Build history of the part. All positions in model axes, mm. A direction names the side the tool comes from. Coordinates: 2 decimals unless noted, no trailing zeros. Write each loop counter-clockwise with the first axis right and the second up, starting at its lowest first coordinate (ties: lowest second). Pieces come first, ordered by that corner, then holes.
from build123d import *

# Parameters (mm, degrees)
BOSS_EXTRUDE1_DEPTH = 6


with BuildPart() as part:
    # Sketch1 → Boss-Extrude1 (new body)
    with BuildSketch(Plane.XY):
        with BuildLine():
            Line((-18.687702572, 18.729195928), (-15.687702572, 18.729195928))
            Line((-15.687702572, 18.729195928), (-15.687702572, 6.729195928))
            Line((-15.687702572, 6.729195928), (-9.687702572, 6.729195928))
            Line((-9.687702572, 6.729195928), (-9.687702572, 12.729195928))
            Line((-9.687702572, 12.729195928), (-6.556235979, 14.903596974))
            ThreePointArc((-6.556235979, 14.903596974), (-2.418100544, 16.566329788), (2.031378501, 16.264698373))
            Line((2.031378501, 16.264698373), (3.503651069, 15.82124278))
            ThreePointArc((3.503651069, 15.82124278), (6.627191746, 15.399192613), (9.726940979, 15.970320798))
            Line((9.726940979, 15.970320798), (14.488027768, 17.656969749))
            Line((14.488027768, 17.656969749), (14.488027768, 4.729195928))
            Line((14.488027768, 4.729195928), (20.488027768, 4.729195928))
            Line((20.488027768, 4.729195928), (20.488027768, 12.729195928))
            Line((20.488027768, 12.729195928), (26.488027768, 12.729195928))
            Line((26.488027768, 12.729195928), (26.488027768, -3.270804072))
            Line((26.488027768, -3.270804072), (3.231231788, -3.270804072))
            Line((3.231231788, -3.270804072), (3.231231788, -9.270804072))
            Line((3.231231788, -9.270804072), (-18.687702572, -9.270804072))
            Line((-18.687702572, -9.270804072), (-18.687702572, 18.729195928))
        make_face()
    extrude(amount=BOSS_EXTRUDE1_DEPTH)


solid = part.part
(1) Slice it at D-D, the plane x = -11. List the corners of the cut face in (y, z), and give its area (3 significant figures).
(2) Slice it at A-A, the plane y = 10.25. List the corners of the cut face in (x, z), and give its area (3 significant figures).
(3) 3-axis set-ups, long thin cutter, end or side, ignore diameter. For faces 4 (the flat face through (26.488, 5, 3)), 5 (the flat face through (-1, 5, 6)), 6 (the flat face through (23, 12.729, 3)), 7 (the flat face through (15, -3.271, 3)), 8 (the flat face through (2.757, 16.046, 2.958)): which of +Z, -Z, +X, -X, +Y, -Y reach the whole face in a straight line?
(4) Flat gauge pins, fed straight in: P1, Ø3, axis at x = 23, z = 3.5, coming from the +Y side; P2, Ø3, axis at x = 18.5, z = 3, coming from the +Y side; P3, Ø1.5, axis at x = 17.5, z = 3, coming from the -Y side. Where does each tip first touch, or does it go through?
(5) Probe L1, parallel to X at y = 12.5, z = 2.2; L2, parallel to X at y = 5.5, z = 1.8; L3, parallel to Y at x = 19.5, z = 5.3. List the from-to ranges inside material, lowest first.
(6) Slice it at C-C, the plane z = 1.6. List the corners of the cut face in (x, y).
(7) Two-plate mould, pull along X, no slides. Class faces 1 (the flat face through (-8, -9.271, 3)), 2 (the flat face through (-18.688, 5, 3)), 3 (the flat face through (-15.688, 13, 3)): pulls with the +X half, pulls with the -X half, needs draft (parallel to the pull), parting line crosses it, or undercut.
(8) Slice it at B-B, the plane y = 13.25. List the corners of the cut face in (x, z).
Results:
1. outline: (-9.27, 0) - (6.73, 0) - (6.73, 6) - (-9.27, 6) - close
1. area: 96.0 mm2
2. outline: (-18.69, 0) - (-15.69, 0) - (-15.69, 6) - (-18.69, 6) - close; (-9.69, 0) - (14.49, 0) - (14.49, 6) - (-9.69, 6) - close; (20.49, 0) - (26.49, 0) - (26.49, 6) - (20.49, 6) - close
2. area: 199 mm2
3. face 4: +Z, -Z, +X, +Y, -Y
3. face 5: +Z, +X, -X, +Y, -Y
3. face 6: +Z, -Z, +X, +Y
3. face 7: +Z, -Z, +X, -Y
3. face 8: +Z, -Z, +Y
4. P1: stops at y = 12.73
4. P2: stops at y = 4.73
4. P3: stops at y = -3.27
5. L1: x = -18.69 to -15.69, -9.69 to 14.49, 20.49 to 26.49
5. L2: x = -18.69 to 14.49, 20.49 to 26.49
5. L3: y = -3.27 to 4.73
6. outline: (-18.69, -9.27) - (3.23, -9.27) - (3.23, -3.27) - (26.49, -3.27) - (26.49, 12.73) - (20.49, 12.73) - (20.49, 4.73) - (14.49, 4.73) - (14.49, 17.66) - (9.73, 15.97) arc R10 cw to (3.5, 15.82) - (2.03, 16.26) arc R10 ccw to (-6.56, 14.9) - (-9.69, 12.73) - (-9.69, 6.73) - (-15.69, 6.73) - (-15.69, 18.73) - (-18.69, 18.73) - close
7. face 1: needs draft
7. face 2: pulls with the -X half
7. face 3: undercut
8. outline: (-18.69, 0) - (-15.69, 0) - (-15.69, 6) - (-18.69, 6) - close; (-8.94, 0) - (14.49, 0) - (14.49, 6) - (-8.94, 6) - close
